Check sheet for the drawn part. Datum: minimum x, y, z corner. Units: mm. Give positions to 0.01 mm unless a question says otherwise; leave off trailing zeros. Order: outer loops, then holes, each group sorted by start corner. A loop starts at its lowest first (then second) coordinate and runs counter-clockwise, first axis right, second up. Notation, with made-up numbers: (0, 1.5) -> (26, 1.5) arc R15 cw to (26, 8.5) -> close; hole circle Ø2 at (57.25, 75). An arc over 180 degrees is marked (long way). One line per question, with ' | ' between items. Start each with the question number.
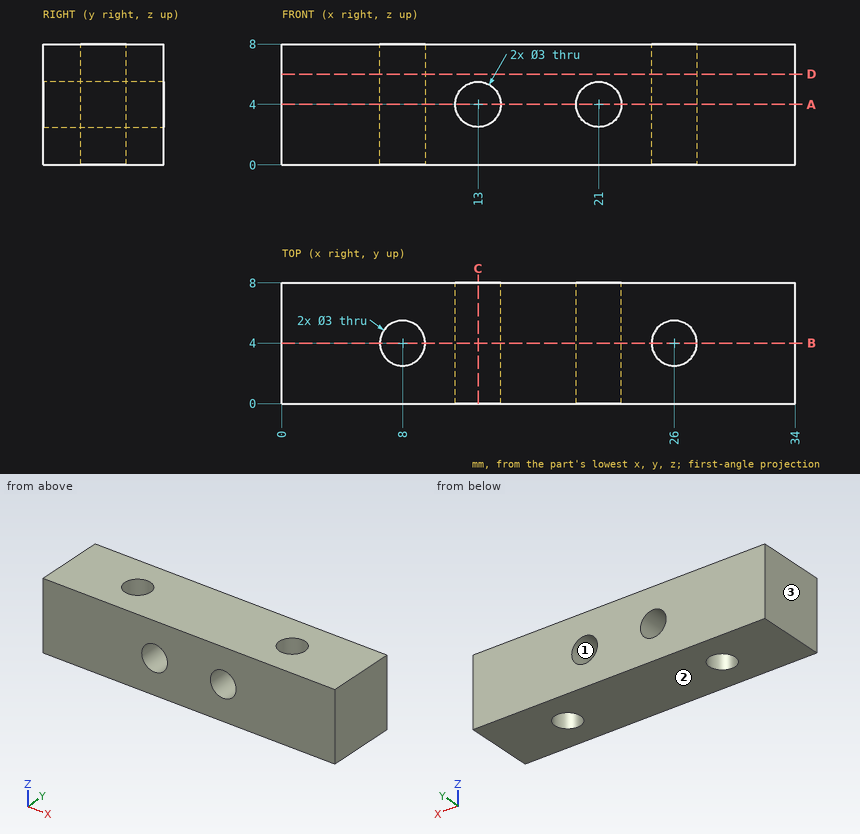
1. Mould release check, pull along X, two halves, no side actions. Record for the marked faces 1, 2 and 3: +X half, -X half, draft (parallel to the pull), parting line (faces both ways), or undercut.
2. Scan lines: probe 1 along X at (y, z) = (6, 4); probe 2 along X at (y, z) = (5.25, 6); probe 3 along Y at (x, z) = (8, 3.75). Record each from-to range of solid material in increasing order.
3. Cross-section at D-D on z = 6. Record the boundary of the cut face in (x, y).
4. Cross-section at A-A on z = 4. Record the boundary of the cut face in (x, y), and give its area (3 significant figures).
5. Cross-section at B-B on y = 4. Record the boundary of the cut face in (x, z), and give its area (3 significant figures).
6. Cross-section at C-C on x = 13. Record the boundary of the cut face in (y, z), and give its area (3 significant figures).
Response values:
1) face 1: undercut | face 2: draft | face 3: -X half
2) probe 1: x = 0 to 11.5, 14.5 to 19.5, 22.5 to 34 | probe 2: x = 0 to 7.17, 8.83 to 25.17, 26.83 to 34 | probe 3: y = 0 to 2.5, 5.5 to 8
3) outline: (0, 0) -> (34, 0) -> (34, 8) -> (0, 8) -> close; hole circle Ø3 at (8, 4); hole circle Ø3 at (26, 4)
4) outline: (0, 0) -> (11.5, 0) -> (11.5, 8) -> (0, 8) -> close; (14.5, 0) -> (19.5, 0) -> (19.5, 8) -> (14.5, 8) -> close; (22.5, 0) -> (34, 0) -> (34, 8) -> (22.5, 8) -> close; hole circle Ø3 at (8, 4); hole circle Ø3 at (26, 4) | area: 210 mm²
5) outline: (0, 0) -> (6.5, 0) -> (6.5, 8) -> (0, 8) -> close; (9.5, 0) -> (24.5, 0) -> (24.5, 8) -> (9.5, 8) -> close; (27.5, 0) -> (34, 0) -> (34, 8) -> (27.5, 8) -> close; hole circle Ø3 at (13, 4); hole circle Ø3 at (21, 4) | area: 210 mm²
6) outline: (0, 0) -> (8, 0) -> (8, 2.5) -> (0, 2.5) -> close; (0, 5.5) -> (8, 5.5) -> (8, 8) -> (0, 8) -> close | area: 40.0 mm²
